Answer from the drawing. Dimensions are ordinates in mm from the lowest x, y and z of the part. Coordinates: 2 decimals unless noted, no trailing zeros. Order: outer loops, then holes, each group sorted by start corner. A loop starts at its lowest first (then second) coordinate and runs counter-clockwise, first axis right, second up. Notation, with made-up numbers: M 8.25,-37 L 22.25,-37 A16 cw 22.25,-17 Z; hole C 35,71 d4. An arc over 180 degrees is marked long. Use a Markdown table: item, result.
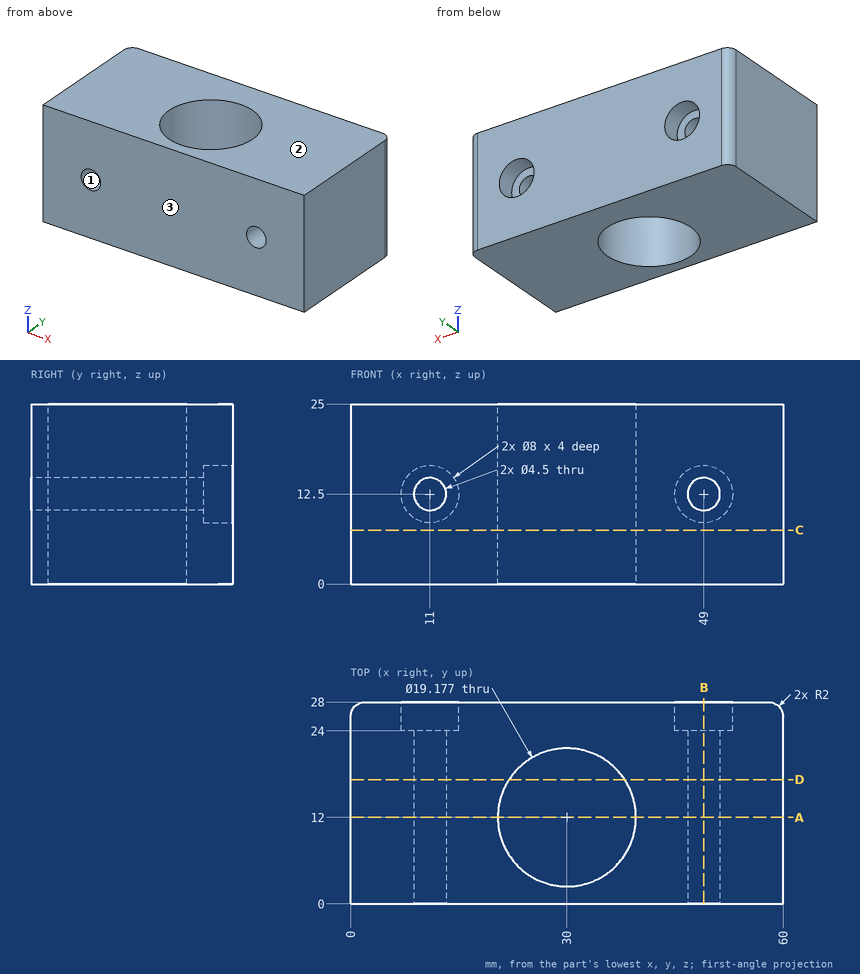
(1) A cutting plane is placed at C-C (z = 7.5). Determine the outline of the cut face in (x, y), then the cut area to 3 significant figures.
Conclusion:
| item | result |
|---|---|
| outline | M 0,0 L 60,0 L 60,26 A2 ccw 58,28 L 2,28 A2 ccw 0,26 Z; hole C 30,12 d19.18 |
| area | 1,390 mm2 |
(2) Given P1, Ø5, axis at y = 20, z = 13, coming from the -X side; P2, Ø6.5, axis at x = 49.5, z = 12, coming from the +Y side, each flat-ended and moving along its own axis, determine where each tip first touches the part or whether it passes through.
Conclusion:
| item | result |
|---|---|
| P1 | x = 0 |
| P2 | y = 24 |
(3) Straight lines are drawn through the part: L1, parallel to Z at x = 11, y = 12.75; L2, parallel to Z at x = 49, y = 26.05; L3, parallel to X at y = 14, z = 14.5. For each, find the intervals that lie inside material, in ascending order.
Conclusion:
| item | result |
|---|---|
| L1 | 0 to 10.25, 14.75 to 25 |
| L2 | 0 to 8.5, 16.5 to 25 |
| L3 | 0 to 9.97, 12.03 to 20.62, 39.38 to 47.97, 50.03 to 60 |
(4) A cutting plane is placed at A-A (y = 12). Determine the outline of the cut face in (x, z), then the cut area to 3 significant figures.
Conclusion:
| item | result |
|---|---|
| outline | M 0,0 L 20.41,0 L 20.41,25 L 0,25 Z; M 39.59,0 L 60,0 L 60,25 L 39.59,25 Z; hole C 11,12.5 d4.5; hole C 49,12.5 d4.5 |
| area | 989 mm2 |
(5) A cutting plane is placed at B-B (x = 49). Determine the outline of the cut face in (y, z).
Conclusion:
| item | result |
|---|---|
| outline | M 0,0 L 28,0 L 28,8.5 L 24,8.5 L 24,10.25 L 0,10.25 Z; M 0,14.75 L 24,14.75 L 24,16.5 L 28,16.5 L 28,25 L 0,25 Z |
(6) Determine the mould class of the marked faces 1, 2 and 3 for opening direction Z: pulls with the +Z half, pulls with the -Z half, needs draft (parallel to the pull), parting line crosses it, or undercut.
Conclusion:
| item | result |
|---|---|
| face 1 | undercut |
| face 2 | pulls with the +Z half |
| face 3 | needs draft |
(7) A cutting plane is placed at D-D (y = 17.25). Determine the outline of the cut face in (x, z).
Conclusion:
| item | result |
|---|---|
| outline | M 0,0 L 21.98,0 L 21.98,25 L 0,25 Z; M 38.02,0 L 60,0 L 60,25 L 38.02,25 Z; hole C 11,12.5 d4.5; hole C 49,12.5 d4.5 |
